from build123d import *

# Parameters (mm, degrees)
F0_W     = 1219.2
F0_H     = 127
F1_DEPTH = 19.05
F2_W     = 18.75663
F2_H     = 25.10663
F3_DEPTH = 19.051
F5_D     = 5


with BuildPart() as f1:
    # F0 (on Front) → F1 (new body)
    with BuildSketch(Plane.XZ):
        Rectangle(F0_W, F0_H)
    extrude(amount=F1_DEPTH)

    # F2 (on face) → F3 (cut, through all)
    with BuildSketch(Plane.XZ.offset(19.05)):
        with Locations((-600.221685, 50.946685)):
            Rectangle(F2_W, F2_H)
        with Locations((600.221685, 50.946685)):
            Rectangle(F2_W, F2_H)
    extrude(amount=-F3_DEPTH, mode=Mode.SUBTRACT)

    # F5 (through all)
    with Locations(Plane.XZ.offset(19.05)):
        with Locations((-514.64337, 51.09337), (-273.34337, 51.09337), (0.29337, 51.09337), (273.34337, 51.09337), (514.64337, 51.09337)):
            Hole(F5_D / 2)


solid = f1.part
CAD build for the part. Positions are in the model's coordinates, mm. A direction names the side the tool comes from. Round coordinates to 2 decimals unless told otherwise and drop trailing zeros. Answer as a JSON object with one key per item and string values.
(1) Pin check, flat tips, straight feed: P1, Ø4.5, axis at x = 514.64, z = 51.09, coming from the +Y side; P2, Ø5.5, axis at y = -9, z = 51, coming from the -X side; P3, Ø5.5, axis at x = 596, y = -12, coming from the +Z side. Stop position of each tip, or through.
Reported:
{"P1": "passes through", "P2": "stops at x = -590.84", "P3": "stops at z = 38.39"}
(2) Which spindle directions (+Z, -Z, +X, -X, +Y, -Y) get a long thin tool onto all of the face, cutting with end or side? Do faces 1 (the face through (-590.843, -10, 51)), 2 (the face through (590.843, -10, 51)), 3 (the face through (609.6, -9, -13)). Say none if no direction does.
Reported:
{"face 1": "+Z, -X, +Y, -Y", "face 2": "+Z, +X, +Y, -Y", "face 3": "+Z, -Z, +X, +Y, -Y"}
(3) Probe probe 1 along X at (y, z) = (-11, 50.5); probe 2 along X at (y, z) = (-13.75, 54). List the from-to ranges inside material, lowest first. Write a range as [from, to].
Reported:
{"probe 1": "x = [-590.84, -517.07], [-512.21, -275.77], [-270.91, -2.14], [2.72, 270.91], [275.77, 512.21], [517.07, 590.84]", "probe 2": "x = [-590.84, 590.84]"}
